Autodesk Inventor part; units mm, degrees
ref_plane "YZ Plane" through (0, 0, 0) normal (1, 0, 0) x (0, 1, 0)
ref_plane "XZ Plane" through (0, 0, 0) normal (0, 1, 0) x (-1, 0, 0)
ref_plane "XY Plane" through (0, 0, 0) normal (0, 0, 1) x (1, 0, 0)
sketch "Sketch6" plane through (0, 0, 0) normal (0, 1, 0) x (-1, 0, 0)
  line L0 (0, 0) -> (-80.4576, 0)
  line L1 (-80.4576, 0) -> (-80.4576, 2980)
  line L2 (-80.4576, 2980) -> (0, 2980)
  line L3 (0, 2980) -> (0, 0)
  dimension "d26" = 80.4576
  dimension "d27" = 2980
extrude "Plate4" add sketch "Sketch6" along normal blind 3
sketch "Sketch9" plane through (0, 3, 0) normal (0, 1, 0) x (1, 0, 0)
  line L0 (0, -2980) -> (0, 0)
  line L1 (80.4576, -2980) -> (0, -2980)
  line L2 (80.4576, 0) -> (80.4576, -2980)
  line L3 (0, 0) -> (80.4576, 0)
  line L4 (25, -2762.0797) -> (10, -2762.0797) construction
  line L5 (10, -2762.0797) -> (10, -2562.0797) construction
  line L6 (10, -2562.0797) -> (25, -2562.0797) construction
  line L7 (25, -2562.0797) -> (25, -2762.0797) construction
  dimension "d44" = 200
  dimension "d45" = 15
  dimension "d47" = 10
mark "Mark1"
sketch "Sketch7" plane through (0, 0, 0) normal (0, -1, 0) x (1, 0, 0)
  line L0 (0, 2980) -> (80.4576, 2980)
  line L1 (0, 0) -> (0, 2980)
  line L2 (80.4576, 0) -> (0, 0)
  line L3 (80.4576, 2980) -> (80.4576, 0)
  line L4 (0, 2798) -> (41.2288, 2798)
  line L5 (41.2288, 2798) -> (41.2288, 2794.8)
  line L6 (41.2288, 2794.8) -> (0, 2794.8)
  line L7 (0, 2794.8) -> (0, 2798)
  point P0 (0, 2794.8)
  point P1 (0, 200)
  point P2 (46.4173, 200)
  point P3 (0, 2794.8)
  dimension "d29" = 41.2288
  dimension "d30" = 3.2
  dimension "d51" = 182
extrude "Extrusion2" cut sketch "Sketch7" against normal through all contours L4 L5 L6 L1
pattern_linear "Rectangular Pattern1" count 6 spacing 500 along (0, 0, -1) of "Extrusion2"
sketch "Sketch8" plane through (0, 0, 0) normal (0, -1, 0) x (1, 0, 0)
  line L0 (0, 2798) -> (41.2288, 2798)
  line L1 (41.2288, 2798) -> (41.2288, 2794.8)
  line L2 (41.2288, 2794.8) -> (0, 2794.8)
  line L3 (0, 0) -> (0, 294.8)
  line L4 (80.4576, 0) -> (0, 0)
  line L5 (80.4576, 2980) -> (80.4576, 0)
  line L6 (0, 2980) -> (80.4576, 2980)
  circle A0 centre (0, 1490) radius 25
  line L7 (0, 2798) -> (0, 2980)
  line L8 (0, 298) -> (41.2288, 298)
  line L9 (41.2288, 298) -> (41.2288, 294.8)
  line L10 (41.2288, 294.8) -> (0, 294.8)
  line L11 (0, 2298) -> (0, 2794.8)
  line L12 (0, 2298) -> (41.2288, 2298)
  line L13 (41.2288, 2298) -> (41.2288, 2294.8)
  line L14 (41.2288, 2294.8) -> (0, 2294.8)
  line L15 (0, 1798) -> (0, 2294.8)
  line L16 (0, 1798) -> (41.2288, 1798)
  line L17 (41.2288, 1798) -> (41.2288, 1794.8)
  line L18 (41.2288, 1794.8) -> (0, 1794.8)
  line L19 (0, 1298) -> (0, 1794.8)
  line L20 (0, 1298) -> (41.2288, 1298)
  line L21 (41.2288, 1298) -> (41.2288, 1294.8)
  line L22 (41.2288, 1294.8) -> (0, 1294.8)
  line L23 (0, 798) -> (0, 1294.8)
  line L24 (0, 798) -> (41.2288, 798)
  line L25 (41.2288, 798) -> (41.2288, 794.8)
  line L26 (41.2288, 794.8) -> (0, 794.8)
  line L27 (0, 298) -> (0, 794.8)
  dimension "d37" = 50
  dimension "d38" = 1490
extrude "Extrusion3" cut sketch "Sketch8" against normal through all contours L19 A0 | A0 L19
pattern_linear "Rectangular Pattern2" count 2 spacing 1480 along (0, 0, 1) of "Extrusion3"
chamfer "Corner Chamfer1" distance 6 angle 45 2 edges at (22.9129, 1.5, 2980) (80.4576, 1.5, 2980)
equation "\"d28\" = Thickness"
equation "\"BendReliefWidth\" = Thickness"
equation "\"BendReliefDepth\" = 0.5 * Thickness"
equation "\"CornerReliefSize\" = 4 * Thickness"
equation "\"MinimumRemnant\" = 2 * Thickness"
equation "\"TransitionRadius\" = BendRadius"
equation "\"JacobiRadiusSize\" = BendRadius"
equation "\"GapSize\" = Thickness"
properties part number "BSH 0341 stringer board 2" material "09g2s"
Here's how the part is built. I have some questions about the finished solid (model axes, mm). Coordinates: 2 decimals unless noted, no trailing zeros. Loops run counter-clockwise (first coordinate to the right, second up) from the corner with the lowest first, then second, coordinate; pieces in that order, holes last.
1. Imagine slicing it at A-A, the plane z = 1490. Please give me the cut outline in (x, y), and give its area (3 significant figures).
2. For P1, Ø0.9, axis at y = 1.5, z = 1296, coming from the -X side, with a flat end and sliding along its axis, tell me the tip position at first contact or that it passes through.
3. I need wall thicknesses on L1, parallel to Z at x = 76, y = 1.95; L2, parallel to X at y = 2.6, z = 1467. Which ranges of each line are inside material? Lowest first, please.
Taken from the geometry:
1. outline: (25, 0) - (80.46, 0) - (80.46, 3) - (25, 3) - close
1. area: 166 mm2
2. P1: stops at x = 41.23
3. L1: z = 0 to 2978.46
3. L2: x = 9.8 to 80.46
